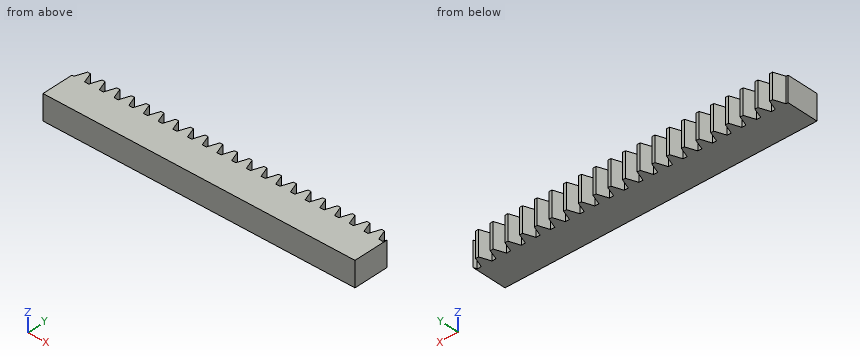
from build123d import *

# Parameters (mm, degrees)
BLANKSKE_W        = 100
BLANKSKE_H        = 13.5
BLANK_DEPTH       = 8
TOOTHCUTSIM_DEPTH = 102.223762032
TEETHCUTS_COUNT   = 22
TEETHCUTS_PITCH   = 4.712388975


with BuildPart() as part:
    # BlankSke → Blank (new body)
    with BuildSketch(Plane.XY):
        with Locations((50, 6.75)):
            Rectangle(BLANKSKE_W, BLANKSKE_H)
    extrude(amount=-BLANK_DEPTH)

    # TooCutSkeSim → ToothCutSim (cut, through all)
    with BuildSketch(Plane.XY):
        Polygon((0.654653055, 10.125), (-0.654653055, 10.125), (-1.892297439, 13.5254), (1.892297439, 13.5254), align=None)
    toothcutsim = extrude(amount=-TOOTHCUTSIM_DEPTH, mode=Mode.SUBTRACT)

    # TeethCuts: ToothCutSim ×22
    with Locations(*[(i * TEETHCUTS_PITCH, 0, 0) for i in range(1, TEETHCUTS_COUNT)]):
        add(toothcutsim, mode=Mode.SUBTRACT)


solid = part.part
Here's how the part is built. I have some questions about the finished solid (model axes, mm). Coordinates: 2 decimals unless noted, no trailing zeros. Answer as CSV lines item,"result". Start each with the question number.
1. I want a section at A-A, the plane y = 12. Count the separate pieces of the cut face and the enclosed holes in it, and give its area (3 significant figures).
2. I need wall thicknesses on line 1 (Y direction, x = 84.5, z = -4) (3 decimals). Which ranges of the line are inside material? Lowest first, please. Write a range as [from, to].
3. For pin 1 (0.7 mm diameter, centred on x = 37.5, z = -5, fed in from +Y) (3 decimals), with a flat end and sliding along its axis, tell me the tip position at first contact or that it passes through.
Recorded:
1,separate pieces,"21"
1,enclosed holes,"0"
1,area,"342 mm2"
2,line 1,"y = [0, 10.125]"
3,pin 1,"stops at y = 10.125"
